from build123d import *

# Parameters (mm, degrees)
F0_R      = 7
F1_DEPTH  = 50
F2_R      = 8
F3_DEPTH  = 2
F4_R      = 7.5
F5_DEPTH  = 46
F6_R      = 6
F7_DEPTH  = 1
F8_R      = 7
F9_DEPTH  = 40
F11_D     = 5
F11_DEPTH = 20
F11_TIP   = 1.5021515476
F13_D     = 5
F13_DEPTH = 20
F13_TIP   = 1.5021515476
F14_SIZE  = 1


with BuildPart() as f1:
    # F0 (on Top) → F1 (new body)
    with BuildSketch(Plane.XY):
        Circle(F0_R)
    extrude(amount=F1_DEPTH)

    # F2 (on face) → F3 (join)
    with BuildSketch(Plane.XY.offset(50)):
        Circle(F2_R)
    extrude(amount=F3_DEPTH)

    # F4 (on face) → F5 (join)
    with BuildSketch(Plane.XY.offset(52)):
        Circle(F4_R)
    extrude(amount=F5_DEPTH)

    # F6 (on face) → F7 (join)
    with BuildSketch(Plane.XY.offset(98)):
        Circle(F6_R)
    extrude(amount=F7_DEPTH)

    # F8 (on face) → F9 (join)
    with BuildSketch(Plane.XY.offset(99)):
        Circle(F8_R)
    extrude(amount=F9_DEPTH)

    # F11
    with Locations(Plane.XY.offset(139)):
        with Locations((0, 0)):
            Hole(F11_D / 2, depth=F11_DEPTH)
            with Locations((0, 0, -(F11_DEPTH + F11_TIP / 2))):  # 118° drill point
                Cone(0, F11_D / 2, F11_TIP, mode=Mode.SUBTRACT)

    # F13
    with Locations(Plane(origin=(0, 0, 0), x_dir=(1, 0, 0), z_dir=(0, 0, -1))):
        with Locations((0, 0)):
            Hole(F13_D / 2, depth=F13_DEPTH)
            with Locations((0, 0, -(F13_DEPTH + F13_TIP / 2))):  # 118° drill point
                Cone(0, F13_D / 2, F13_TIP, mode=Mode.SUBTRACT)

    # F14
    f14_edges = [f1.edges().sort_by_distance(p)[0] for p in [
        (-7, 0, 0),
        (-7, 0, 139),
        (-7.5, 0, 98),
    ]]
    chamfer(f14_edges, length=F14_SIZE)


solid = f1.part
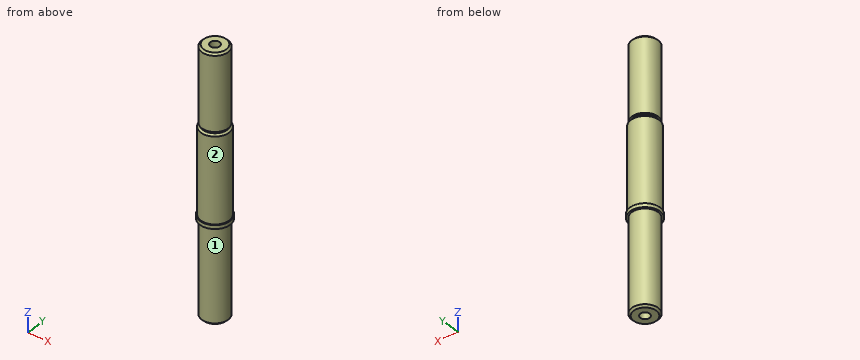
Build history of the part. All positions in model axes, mm. Face numbers are marked on the shaded views. A direction names the side the tool comes from. Coordinates: 2 decimals unless noted, no trailing zeros. Write each loop counter-clockwise with the first axis right and the second up, starting at its lowest first coordinate (ties: lowest second). Pieces come first, ordered by that corner, then holes.
(1) Cut at B-B on z = 84.5. List the corners of the cut face in (x, y), and give its area (3 significant figures).
(2) Drill centre lines: line 1 (Y direction, x = -0.25, z = 105.5); line 2 (Y direction, x = 0, z = 10.25); line 3 (Y direction, x = -4.5, z = 95). Where is each one in solid material? Low to high.
(3) Pin check, flat tips, straight feed: pin 1 Ø6 at (y, z) = (3, 90.5) entering from +X; pin 2 Ø5 at (x, z) = (1.5, 87) entering from +Y; pin 3 Ø3 at (x, z) = (-5, 77.5) entering from -Y. Stop position of each tip, or through.
(4) 3-axis set-ups, long thin cutter, end or side, ignore diameter. For the marked faces 1 and 2: which of +Z, -Z, +X, -X, +Y, -Y reach the whole face in a straight line?
(5) Cut at A-A on z = 122. List the corners of the cut face in (x, y), and give its area (3 significant figures).
Working result:
1. outline: circle Ø15 at (0, 0)
1. area: 177 mm2
2. line 1: y = -7 to 7
2. line 2: y = -7 to -2.5, 2.5 to 7
2. line 3: y = -6 to 6
3. pin 1: stops at x = 7.5
3. pin 2: stops at y = 7.5
3. pin 3: stops at y = -6.63
4. face 1: -Z
4. face 2: +Z
5. outline: circle Ø14 at (0, 0); hole circle Ø5 at (0, 0)
5. area: 134 mm2
